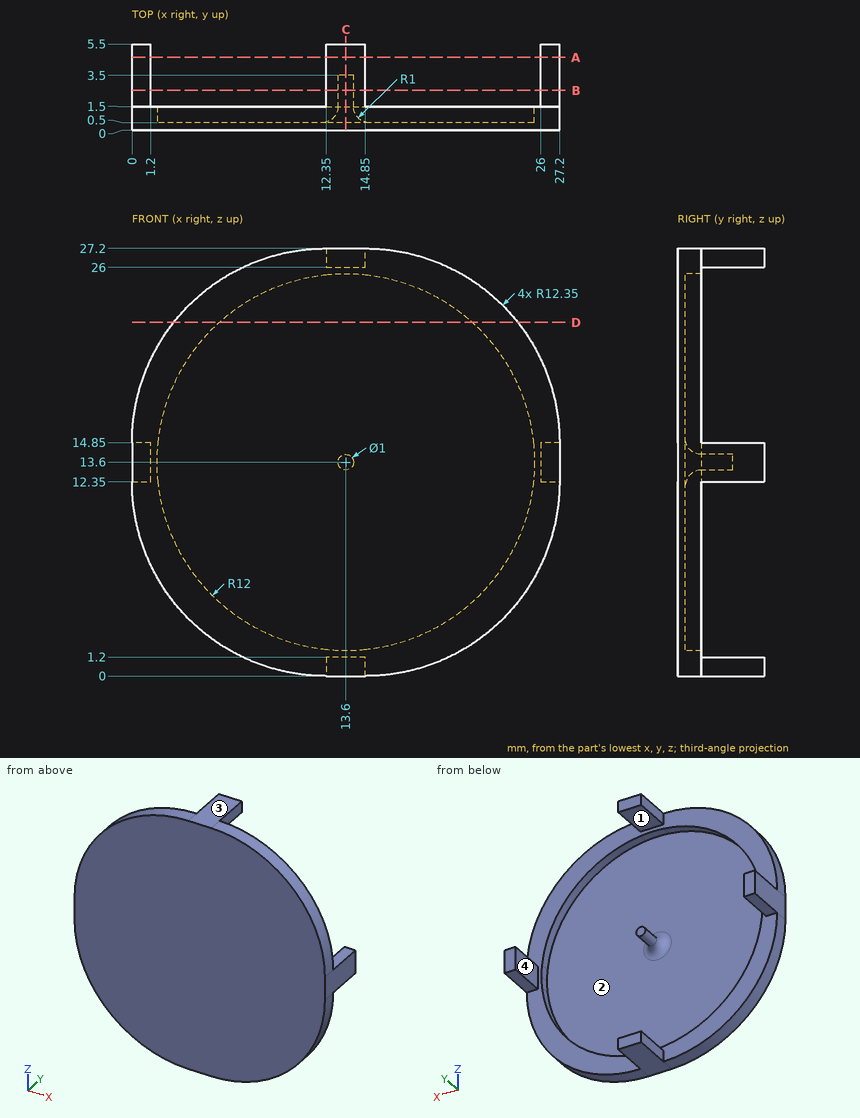
Geometry check sheet. Reference: drawing and pictorial views, mm from the part's lowest x, y, z. A direction names the side the tool comes from. Round coordinates to 2 decimals unless told otherwise and drop trailing zeros. Loops run counter-clockwise (first coordinate to the right, second up) from the corner with the lowest first, then second, coordinate; pieces in that order, holes last. Notation, with made-up numbers: (-6, 15.5) - (26, 15.5) arc R27 ccw to (26, 54.5) - close; hole circle Ø9 at (63.25, 58). An arc over 180 degrees is marked (long way). One line per question, with ' | ' between items. Start each with the question number.
1. Tool access check on the marked faces 1, 2, 3 and 4. Record the directions out of +Z, -Z, +X, -X, +Y, -Y that give a thin tool (end or side, any length) a straight path to the whole face; none if there is none.
2. Cross-section at D-D on z = 22.5. Record the cut outline in (x, y), then the cut area to 3 significant figures.
3. Scan lines: line 1 (Y direction, x = 3, z = 12.75); line 2 (Y direction, x = 22.75, z = 3.75); line 3 (X direction, y = 0.6, z = 11.5). Record each from-to range of solid material in increasing order. Write a range as [from, to].
4. Depth check by flat-ended pin: pin 1 (0.6 mm diameter, centred on x = 27, y = 2.5, fed in from -Z); pin 2 (3 mm diameter, centred on x = 5.5, z = 23, fed in from +Y); pin 3 (0.6 mm diameter, centred on x = 26.5, y = 2.5, fed in from +Z); pin 4 (0.8 mm diameter, centred on y = 4.5, z = 13.5, fed in from -X). Enter the tip coordinate at first touch or a pass-through.
5. Cross-section at A-A on y = 4.65. Record the cut outline in (x, z).
6. Cross-section at B-B on y = 2.55. Record the cut outline in (x, z).
7. Cross-section at C-C on x = 13.6. Record the cut outline in (y, z).
Taken from the geometry:
1) face 1: +X, -X, +Y | face 2: +Y | face 3: +Z, +X, -X, +Y, -Y | face 4: +Z, -Z, +Y
2) outline: (2.65, 0) - (24.55, 0) - (24.55, 1.5) - (21.65, 1.5) - (21.65, 0.5) - (5.55, 0.5) - (5.55, 1.5) - (2.65, 1.5) - close | area: 16.7 mm²
3) line 1: [0, 0.5] | line 2: [0, 1.5] | line 3: [0.03, 1.79], [25.41, 27.17]
4) pin 1: z = 12.35 | pin 2: y = 1.5 | pin 3: z = 14.85 | pin 4: x = 0
5) outline: (0, 12.35) - (1.2, 12.35) - (1.2, 14.85) - (0, 14.85) - close; (12.35, 0) - (14.85, 0) - (14.85, 1.2) - (12.35, 1.2) - close; (12.35, 26) - (14.85, 26) - (14.85, 27.2) - (12.35, 27.2) - close; (26, 12.35) - (27.2, 12.35) - (27.2, 14.85) - (26, 14.85) - close
6) outline: (0, 12.35) - (1.2, 12.35) - (1.2, 14.85) - (0, 14.85) - close; (12.35, 0) - (14.85, 0) - (14.85, 1.2) - (12.35, 1.2) - close; (12.35, 26) - (14.85, 26) - (14.85, 27.2) - (12.35, 27.2) - close; circle Ø1 at (13.6, 13.6); (26, 12.35) - (27.2, 12.35) - (27.2, 14.85) - (26, 14.85) - close
7) outline: (0, 0) - (5.5, 0) - (5.5, 1.2) - (1.5, 1.2) - (1.5, 1.6) - (0.5, 1.6) - (0.5, 12.1) arc R1 cw to (1.5, 13.1) - (3.5, 13.1) - (3.5, 14.1) - (1.5, 14.1) arc R1 cw to (0.5, 15.1) - (0.5, 25.6) - (1.5, 25.6) - (1.5, 26) - (5.5, 26) - (5.5, 27.2) - (0, 27.2) - close
